Check sheet for the modelled part. Datum: model origin and axes. Units: mm. A direction names the side the tool comes from. Round coordinates to 2 decimals unless told otherwise and drop trailing zeros. Loops run counter-clockwise (first coordinate to the right, second up) from the corner with the lowest first, then second, coordinate; pieces in that order, holes last. Notation, with made-up numbers: (-9, 1) - (0, 1) arc R8 ccw to (0, 16) - close; hole circle Ø6 at (14, -32). An arc over 180 degrees is marked (long way). Put each result on its own line as item: value. Start each with the question number.
Item 1: Section check B-B, the plane z = 24. Record the cut outline in (x, y), and give its area (3 significant figures).
Item 2: Material ranges on line 1 along X through (y, z) = (13, 42); line 2 along X through (y, z) = (9, 20); line 3 along X through (y, z) = (31.5, 29), recorded low to high.
Item 3: Section check A-A, the plane y = 5. Record the cut outline in (x, z).
Item 4: Tool access check on faces 1 (the flat face through (-16.19, 17.86, 36.17)), 2 (the flat face through (0.24, 43.46, 50.28)). Record the directions out of +Z, -Z, +X, -X, +Y, -Y that give a thin tool (end or side, any length) a straight path to the whole face; none if there is none.
Item 5: Draft check along X on faces 3 (the flat face through (-2, 32, 0)), 4 (the flat face through (-33.785, 17.502, 44.982)), 5 (the flat face through (33.788, 25.315, 36.167)). Enter one of: pulls with the +X half, pulls with the -X half, needs draft (parallel to the pull), parting line crosses it, or undercut.
Item 6: Gauge pin test, flat ends, axial feed: pin 1 Ø2 at (y, z) = (32.5, 68.5) entering from -X; pin 2 Ø3 at (x, z) = (2, 78.5) entering from +Y; pin 3 Ø8 at (y, z) = (39, 70.5) entering from +X. Record the tip position at first contact, or that the pin passes through.
Item 7: Section check C-C, the plane y = 18. Record the cut outline in (x, z).
Item 8: Section check D-D, the plane x = 18. Record the cut outline in (y, z).
from build123d import *


with BuildPart() as f3:
    # F0 (on Top) → F3 section 0
    with BuildSketch(Plane.XY, mode=Mode.PRIVATE) as f3_s0:
        Polygon((58.2950860262, 54.6516403556), (-59.4609826803, 54.6516403556), (-59.4657808542, 0), (-43.416608125, 26.23029612), (-32.3482118547, 0), (-12.4250994995, 28.4439753741), (0, 0), (26.0375738144, 28.7206843495), (38.7662313879, 0), align=None)
    loft([f3_s0.sketch, Vertex(-1.0539550567, 26.3785235584, 127)])


solid = f3.part
Check result:
1. outline: (-48.43, 4.98) - (-35.41, 26.26) - (-26.43, 4.98) - (-10.28, 28.05) - (-0.2, 4.98) - (20.92, 28.28) - (31.24, 4.98) - (47.08, 49.31) - (-48.42, 49.31) - close
1. area: 2,980 mm²
2. line 1: -40.15 to -37.53, -23.8 to -19, -2.22 to 3.53, 23.7 to 27.13
2. line 2: -50.27 to -47.3, -29.46 to -24.03, -2.28 to 4.23, 30.35 to 34.23
2. line 3: -46.13 to 38.78
3. outline: (-59.47, 0) - (-56.41, 0) - (-48.39, 24.07) - close; (-34.46, 0) - (-28.85, 0) - (-26.42, 24.07) - close; (-2.18, 0) - (4.53, 0) - (-0.2, 24.07) - close; (31.22, 24.07) - (36.55, 0) - (40.55, 0) - close
4. face 1: -Y
4. face 2: +Z, +X, -X, +Y
5. face 3: needs draft
5. face 4: undercut
5. face 5: pulls with the +X half
6. pin 1: x = -28.42
6. pin 2: y = 37.51
6. pin 3: x = 27.18
7. outline: (-59.46, 0) - (-48.45, 0) - (-19.61, 86.66) - close; (-39.94, 0) - (-19.74, 0) - (-10.99, 86.66) - close; (-7.86, 0) - (16.32, 0) - (-0.72, 86.66) - close; (11.59, 86.66) - (30.79, 0) - (45.2, 0) - close
8. outline: (13.76, 66.23) - (28.03, 37.68) - (19.85, 0) - (54.65, 0) - (35.46, 86.23) - close
